Study the drawing (mm; zero at the part's minimum x, y, z) and answer. Round coordinates to 2 decimals unless told otherwise and drop trailing zeros. Order: outer loops, then holes, each group sorted by start corner. A loop starts at its lowest first (then second) coordinate and runs counter-clockwise, first axis right, second up. Notation, with made-up numbers: (-19.75, -40) - (-7.75, -40) arc R30 cw to (-7.75, -12) - close; hole circle Ø1 at (52, 78). An arc over 180 degrees is marked (long way). Use one line per item in the form item = value. Start each with the question number.
Q1. Find the intervals of material crossed by line 1 (Y direction, x = 9.25, z = 0.15); line 2 (X direction, y = 9.5, z = 0.2) (1 decimal); line 3 (Y direction, x = 7.5, z = 0.05) (1 decimal), in increasing order. Write a range as [from, to].
Q2. Given P1, Ø1, axis at x = 5.5, y = 6, coming from the -Z side, flat-ended and moving along its own axis, determine where the tip first touches the part or whether it passes through.
Q3. The part is cut by section B-B on z = 0.15. Determine the outline of the cut face in (x, y).
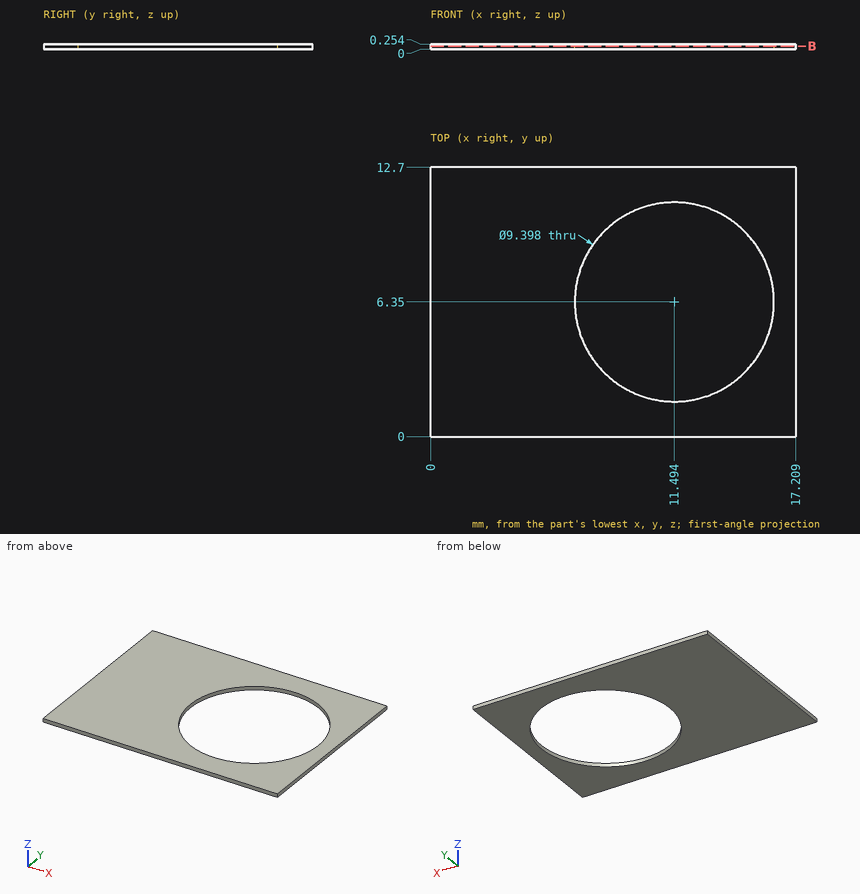
Found:
q1.line_1 = [0, 2.22], [10.48, 12.7]
q1.line_2 = [0, 8], [15, 17.2]
q1.line_3 = [0, 3.9], [8.8, 12.7]
q2.P1 = 0
q3.outline = (0, 0) - (17.21, 0) - (17.21, 12.7) - (0, 12.7) - close; hole circle Ø9.4 at (11.49, 6.35)
